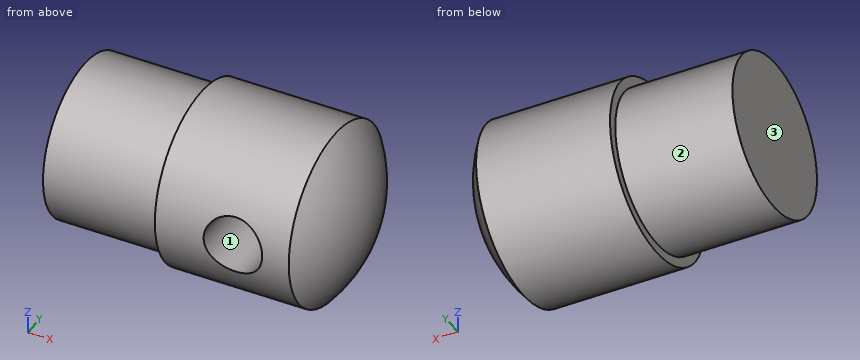
```python
from build123d import *


with BuildPart() as part:
    # Esquisse1 → Révolution1 (revolve)
    with BuildSketch(Plane.XY, mode=Mode.PRIVATE) as r_volution1_sk:
        with BuildLine():
            Line((-117.412392243, 9), (-103.688586948, 9))
            ThreePointArc((-103.688586948, 9), (-101.256912887, 4.78887909), (-100.412392243, 0))
            Line((-100.412392243, 0), (-129.412392243, 0))
            Line((-129.412392243, 0), (-129.412392243, 8))
            Line((-129.412392243, 8), (-117.412392243, 8))
            Line((-117.412392243, 8), (-117.412392243, 9))
        make_face()
    revolve(r_volution1_sk.sketch.rotate(Axis((-129.412392243, 0, 0), (1, 0, 0)), 90), axis=Axis((-129.412392243, 0, 0), (1, 0, 0)))  # turned: the seam where the file's is

    # Esquisse2 → Enlèvement de matière-Révolution1 (revolve, cut)
    with BuildSketch(Plane.XY, mode=Mode.PRIVATE) as enl_vement_de_mati_re_r_volution1_sk:
        with BuildLine():
            Line((-109.412392243, -10.843650203), (-106.412392243, -10.843650203))
            Line((-106.412392243, -10.843650203), (-106.412392243, 0))
            ThreePointArc((-106.412392243, 0), (-107.291071899, 2.121320344), (-109.412392243, 3))
            Line((-109.412392243, 3), (-109.412392243, 0))
            Line((-109.412392243, 0), (-109.412392243, -10.843650203))
        make_face()
    revolve(enl_vement_de_mati_re_r_volution1_sk.sketch.rotate(Axis((-109.412392243, 10.689425153, 0), (0, -1, 0)), 90), axis=Axis((-109.412392243, 10.689425153, 0), (0, -1, 0)), mode=Mode.SUBTRACT)  # turned: the seam where the file's is


solid = part.part
```
Source: CAD feature listing. Evaluate the final solid. Frame: model axes, mm. Face numbers are marked on the shaded views. Give positions to 0.01 mm unless a question says otherwise; leave off trailing zeros. Loops run counter-clockwise (first coordinate to the right, second up) from the corner with the lowest first, then second, coordinate; pieces in that order, holes last. Notation, with made-up numbers: (67, 27.5) -> (109, 27.5) arc R6 ccw to (109, 34.5) -> close; hole circle Ø2 at (17.25, 72). An arc over 180 degrees is marked (long way). Use a Markdown table: item, result. Add a question column.
(1) Section query A-A (z = 0). Output: boundary loops of the cut face in (x, y), then the cut area to 3 significant figures.
(2) Section query C-C (x = -104.75). Output: boundary loops of the cut face in (y, z).
(3) Section query D-D (y = 5.25). Output: boundary loops of the cut face in (x, z).
(4) Pull-direction query (X, two-part tool) for the marked faces 1, 2 and 3; classes: +X half, -X half, draft (parallel to the pull), parting line (faces both ways), or undercut.
(5) Ray query, line 1 (X direction, y = -4.25, z = 0); line 2 (X direction, y = -6.75, z = 0); line 3 (Z direction, x = -109, y = 2.5). Return the intervals inside material, ascending.
(6) Section query B-B (y = -6.75). Output: boundary loops of the cut face in (x, z).
(7) First-contact query: pin 1 Ø2 at (y, z) = (-3, -4.5) entering from +X; pin 2 Ø10 at (x, y) = (-111, -4) entering from +Z; pin 3 Ø5 at (x, y) = (-118, -5) entering from -Z; pin 4 Ø1 at (y, z) = (-1, -1) entering from +X. Flat tips, straight axial feed; report the tip coordinate or a pass-through.
Checked values:
| question | item | result |
|---|---|---|
| 1 | outline | (-129.41, -8) -> (-117.41, -8) -> (-117.41, -9) -> (-112.41, -9) -> (-112.41, 0) arc R3 cw to (-106.41, 0) -> (-106.41, -9) -> (-103.69, -9) arc R14 ccw to (-103.69, 9) -> (-117.41, 9) -> (-117.41, 8) -> (-129.41, 8) -> close |
| 1 | area | 411 mm^2 |
| 2 | outline | circle Ø18 at (0, 0) |
| 3 | outline | (-129.41, -6.04) -> (-117.41, -6.04) -> (-117.41, -7.31) -> (-103.69, -7.31) arc R12.98 ccw to (-103.69, 7.31) -> (-117.41, 7.31) -> (-117.41, 6.04) -> (-129.41, 6.04) -> close |
| 4 | face 1 | undercut |
| 4 | face 2 | draft |
| 4 | face 3 | -X half |
| 5 | line 1 | -129.41 to -112.41, -106.41 to -101.07 |
| 5 | line 2 | -129.41 to -112.41, -106.41 to -102.15 |
| 5 | line 3 | -8.65 to -1.61, 1.61 to 8.65 |
| 6 | outline | (-129.41, -4.29) -> (-117.41, -4.29) -> (-117.41, -5.95) -> (-103.69, -5.95) arc R12.27 ccw to (-103.69, 5.95) -> (-117.41, 5.95) -> (-117.41, 4.29) -> (-129.41, 4.29) -> close; hole circle Ø6 at (-109.41, 0) |
| 7 | pin 1 | x = -101.12 |
| 7 | pin 2 | z = 9 |
| 7 | pin 3 | z = -8.63 |
| 7 | pin 4 | x = -100.44 |
